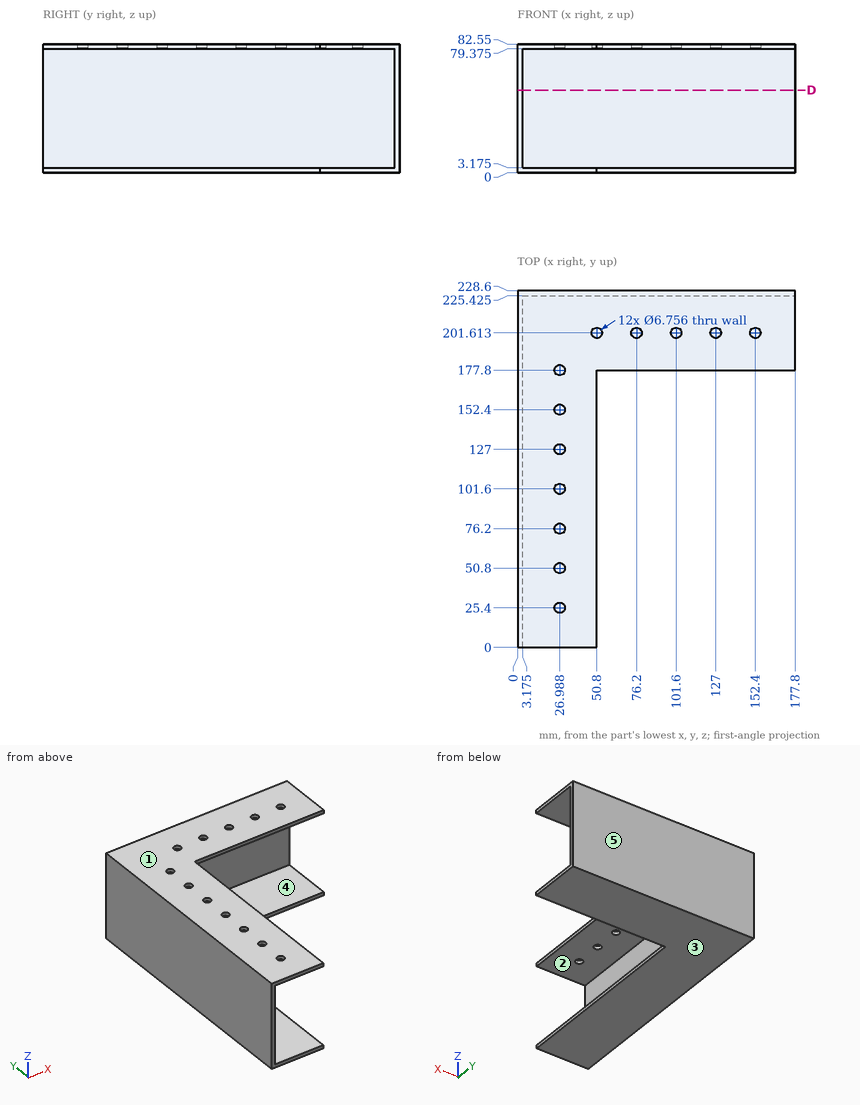
The figure shows three views and two pictorial views of one solid part (mm, origin at its lowest corner). Answer the questions. A direction names the side the tool comes from. Coordinates: 2 decimals unless noted, no trailing zeros. Order: outer loops, then holes, each group sorted by start corner. A loop starts at its lowest first (then second) coordinate and runs counter-clockwise, first axis right, second up. Notation, with made-up numbers: M 2,-3 L 8,-3 A16 ccw 8,2 Z; hole C 44,71 d4. An arc over 180 degrees is marked long. Use CSV: the item, a comma, the result in double quotes.
1) Consider line 1 (Y direction, x = 152.4, z = 80) (1 decimal); line 2 (X direction, y = 25, z = 80); line 3 (X direction, y = 143.5, z = 51) (1 decimal). Determine where each line is inside the solid, lowest interval first. Write a range as [from, to].
Worked out:
line 1,"y = [177.8, 198.2], [205, 228.6]"
line 2,"x = [0, 23.63], [30.34, 50.8]"
line 3,"x = [0, 3.2]"
2) For the marked faces 1 and 2, determine the directions among +Z, -Z, +X, -X, +Y, -Y from which every point of the face is accessible in a straight line to the end or side of a thin tool.
Worked out:
face 1,"+Z, +X, -X, +Y, -Y"
face 2,"+X, -Y"
3) Flat-ended cylindrical pins translate along their axes: pin 1 Ø2 at (x, z) = (25.5, 33) entering from -Y (1 decimal); pin 2 Ø5.5 at (x, y) = (50.8, 201.61) entering from +Z (1 decimal); pin 3 Ø6 at (y, z) = (45.5, 48) entering from +X (1 decimal). Find the tip coordinate at first contact, or state that the pin passes through.
Worked out:
pin 1,"stops at y = 225.4"
pin 2,"stops at z = 3.2"
pin 3,"stops at x = 3.2"
4) Section D-D on z = 53 is taken. Write down the section's boundary in (x, y) (1 decimal).
Worked out:
outline,"M 0,0 L 3.2,0 L 3.2,225.4 L 177.8,225.4 L 177.8,228.6 L 0,228.6 Z"
5) Determine the mould class of the marked faces 3, 4 and 5 for opening direction Z: released by +Z, released by -Z, zero draft, split by the parting line, or undercut.
Worked out:
face 3,"released by -Z"
face 4,"undercut"
face 5,"zero draft"
